```python
from build123d import *

# Parameters (mm, degrees)
F0_W     = 150
F0_H     = 5
F1_DEPTH = 60
F2_W     = 5
F2_H     = 5
F3_DEPTH = 5
F4_R     = 1.75
F4_W     = 5
F4_H     = 5
F5_DEPTH = 5


with BuildPart() as f1:
    # F0 (on Top) → F1 (new body)
    with BuildSketch(Plane.XY):
        with Locations((75, 2.5)):
            Rectangle(F0_W, F0_H)
    extrude(amount=F1_DEPTH)

    # F2 (on face) → F3 (join, through all)
    with BuildSketch(Plane.XZ):
        with Locations((17.5, -2.5)):
            Rectangle(F2_W, F2_H)
        with Locations((42.5, -2.5)):
            Rectangle(F2_W, F2_H)
        with Locations((107.5, -2.5)):
            Rectangle(F2_W, F2_H)
        with Locations((132.5, -2.5)):
            Rectangle(F2_W, F2_H)
        with Locations((42.5, 62.5)):
            Rectangle(F2_W, F2_H)
        with Locations((17.5, 62.5)):
            Rectangle(F2_W, F2_H)
        with Locations((132.5, 62.5)):
            Rectangle(F2_W, F2_H)
        with Locations((107.5, 62.5)):
            Rectangle(F2_W, F2_H)
    extrude(amount=-F3_DEPTH)

    # F4 (on face) → F5 (cut, through all)
    with BuildSketch(Plane.XZ):
        Polygon((28.5, 2), (28.5, 0), (31.5, 0), (31.5, 2), (32.75, 2), (32.75, 5), (31.5, 5), (31.5, 6), (28.5, 6), (28.5, 5), (27.25, 5), (27.25, 2), align=None)
        Polygon((118.5, 6), (118.5, 5), (117.25, 5), (117.25, 2), (118.5, 2), (118.5, 0), (121.5, 0), (121.5, 2), (122.75, 2), (122.75, 5), (121.5, 5), (121.5, 6), align=None)
        Polygon((121.5, 55), (122.75, 55), (122.75, 58), (121.5, 58), (121.5, 60), (118.5, 60), (118.5, 58), (117.25, 58), (117.25, 55), (118.5, 55), (118.5, 54), (121.5, 54), align=None)
        Polygon((31.5, 54), (31.5, 55), (32.75, 55), (32.75, 58), (31.5, 58), (31.5, 60), (28.5, 60), (28.5, 58), (27.25, 58), (27.25, 55), (28.5, 55), (28.5, 54), align=None)
        with Locations((2.5, 30)):
            Circle(F4_R)
        with Locations((2.5, 42.5)):
            Rectangle(F4_W, F4_H)
        with Locations((2.5, 17.5)):
            Rectangle(F4_W, F4_H)
        with Locations((147.5, 42.5)):
            Rectangle(F4_W, F4_H)
        with Locations((147.5, 30)):
            Circle(F4_R)
        with Locations((147.5, 17.5)):
            Rectangle(F4_W, F4_H)
    extrude(amount=-F5_DEPTH, mode=Mode.SUBTRACT)


solid = f1.part
```
Model file for the job. Use its own axes, mm. A direction names the side the tool comes from. Give positions to 0.01 mm unless a question says otherwise; leave off trailing zeros. Order: outer loops, then holes, each group sorted by start corner. A loop starts at its lowest first (then second) coordinate and runs counter-clockwise, first axis right, second up.
1) Saw through at B-B, the plane z = 18. Write the cut outline in (x, y), then the cut area to 3 significant figures.
2) 3-axis set-ups, long thin cutter, end or side, ignore diameter. For faces 4 (the flat face through (7, 3, 60)), 5 (the flat face through (45, 2, 62)), 6 (the flat face through (150, 2, 30)), 7 (the flat face through (36, 3, 0)), 8 (the flat face through (142, 3, 0)): which of +Z, -Z, +X, -X, +Y, -Y reach the whole face in a straight line?
3) Wall check: probe 1 along Z at (x, y) = (147.5, 3.2); probe 2 along Z at (x, y) = (27.5, 0.55); probe 3 along X at (y, z) = (1.35, 29.5). Give the ranges that are in metal, low to high.
4) Saw through at A-A, the plane x = 2.5. Write the cut outline in (y, z).
5) Mould opens along Z. For faces 1 (the flat face through (24, 3, 0)), 2 (the flat face through (32.75, 2, 3)), 3 (the flat face through (17, 2, 65)) say: +Z half, -Z half, draft (parallel to the pull), parting line (faces both ways), or undercut.
6) Saw through at D-D, the plane x = 69.5. Write the cut outline in (y, z), then the cut area to 3 significant figures.
7) Saw through at C-C, the plane y = 3.6. Count the separate pieces of the cut face and the enclosed holes in it, then the cut area to 3 significant figures.
8) Pin check, flat tips, straight feed: pin 1 (2 mm diameter, centred on y = 1, z = 5.5, fed in from -X); pin 2 (0.6 mm diameter, centred on x = 118, y = 3, fed in from +Z); pin 3 (1.5 mm diameter, centred on y = 3.5, z = -2, fed in from -X); pin 4 (1.5 mm diameter, centred on y = 3.5, z = 18.5, fed in from -X). Stop position of each tip, or through.
Computed:
1. outline: (5, 0) - (145, 0) - (145, 5) - (5, 5) - close
1. area: 700 mm2
2. face 4: +Z, -X, +Y, -Y
2. face 5: +Z, +Y, -Y
2. face 6: +Z, -Z, +X, +Y, -Y
2. face 7: -Z, +Y, -Y
2. face 8: -Z, +X, +Y, -Y
3. probe 1: z = 0 to 15, 20 to 28.25, 31.75 to 40, 45 to 60
3. probe 2: z = 0 to 2, 5 to 55, 58 to 60
3. probe 3: x = 0 to 0.82, 4.18 to 145.82, 149.18 to 150
4. outline: (0, 0) - (5, 0) - (5, 15) - (0, 15) - close; (0, 20) - (5, 20) - (5, 28.25) - (0, 28.25) - close; (0, 31.75) - (5, 31.75) - (5, 40) - (0, 40) - close; (0, 45) - (5, 45) - (5, 60) - (0, 60) - close
5. face 1: -Z half
5. face 2: undercut
5. face 3: +Z half
6. outline: (0, 0) - (5, 0) - (5, 60) - (0, 60) - close
6. area: 300 mm2
7. separate pieces: 1
7. enclosed holes: 2
7. area: 8,980 mm2
8. pin 1: stops at x = 0
8. pin 2: stops at z = 60
8. pin 3: stops at x = 15
8. pin 4: stops at x = 5
